from build123d import *

# Parameters (mm, degrees)
F1_DEPTH         = 17.5
F2_W             = 8
F2_H             = 3
F2_W_2           = 15
F2_H_2           = 1
F3_DEPTH         = 50
F5_DEPTH         = 2.5
F5_COPIES2_COUNT = 2


# Not quite as in the source:
# - a pattern or mirror of a feature is missing from the dataset's text; its kind, count and spacing are read off the source's solid


with BuildPart() as f1:
    # F0 (on Front) → F1 (new body, symmetric)
    with BuildSketch(Plane.XZ):
        Polygon((-11.8, 0), (0, 0), (11.8, 0), (11.8, 8), (11.5, 8), (8.5, 2.5), (0, 2.5), (-8.5, 2.5), (-11.5, 8), (-11.8, 8), align=None)
    extrude(amount=F1_DEPTH, both=True)

    # F2 (on Right) → F3 (cut, symmetric)
    with BuildSketch(Plane.YZ):
        with Locations((0, 4)):
            Rectangle(F2_W, F2_H)
        with Locations((0, 0.5)):
            Rectangle(F2_W_2, F2_H_2)
    extrude(amount=F3_DEPTH, both=True, mode=Mode.SUBTRACT)

    # F4 (on Top) → F5 (join)
    with BuildSketch(Plane.XY):
        Polygon((16, 18.5), (11.8, 17.5), (11.8, 7.5), (20, 15.5), (20, 31.5), (16, 31.5), align=None)
    f5 = extrude(amount=F5_DEPTH)

    # F5_copies: F5 across plane
    add(f5.mirror(Plane(origin=(0, 0, 0), x_dir=(0, 0, -1), z_dir=(-1, 0, 0))))

    # F5_copies1: F5 across plane
    add(f5.mirror(Plane(origin=(0, 0, 0), x_dir=(0, 0, -1), z_dir=(0, -1, 0))))

    # F5_copies2: F5 ×2 about axis
    f5_copies2_axis = Axis((0, 0, 0), (0, 0, 1))
    for i in range(1, F5_COPIES2_COUNT):
        add(f5.rotate(f5_copies2_axis, i * 360 / F5_COPIES2_COUNT))


solid = f1.part
Input: part model. Units: mm. Frame: model coordinates. A direction names the side the tool comes from. Give positions to 0.01 mm unless a question says otherwise; leave off trailing zeros. Order: outer loops, then holes, each group sorted by start corner. A loop starts at its lowest first (then second) coordinate and runs counter-clockwise, first axis right, second up. Notation, with made-up numbers: M -7,87 L 12,87 A18 ccw 12,107 Z; hole C 61,44.25 d8. An arc over 180 degrees is marked long. Answer as a JSON object with one key per item and string values.
1. Pull-direction query (Z, two-part tool) for faces 1 (the flat face through (18, 31.5, 1)), 2 (the flat face through (0, -17, 0)), 3 (the flat face through (10, 4, 4)); classes: +Z half, -Z half, draft (parallel to the pull), parting line (faces both ways), or undercut.
Result sheet:
{"face 1": "draft", "face 2": "-Z half", "face 3": "undercut"}
2. Cut plane A-A, the plane y = -26. Output: boundary loops of the cut face in (x, z), and give its area (3 significant figures).
Result sheet:
{"outline": "M -20,0 L -16,0 L -16,2.5 L -20,2.5 Z; M 16,0 L 20,0 L 20,2.5 L 16,2.5 Z", "area": "20.0 mm²"}
3. Cut plane B-B, the plane x = -14.5. Output: boundary loops of the cut face in (y, z), and give its area (3 significant figures).
Result sheet:
{"outline": "M -18.14,0 L -10.13,0 L -10.13,2.5 L -18.14,2.5 Z; M 10.13,0 L 18.14,0 L 18.14,2.5 L 10.13,2.5 Z", "area": "40.0 mm²"}
4. Reachability of faces 4 (the flat face through (17, 20, 2.5)), 5 (the flat face through (-17, -20, 2.5)), 6 (the flat face through (16, -25, 1)), 7 (the flat face through (-11, 4, 4)), 8 (the flat face through (13.9, 18, 1.2)) from +Z, -Z, +X, -X, +Y, -Y: full face, straight path, thin tool, end or side. Return the list, or none.
Result sheet:
{"face 4": "+Z, +X, +Y, -Y", "face 5": "+Z, -X, +Y, -Y", "face 6": "+Z, -Z, -Y", "face 7": "+X, -X", "face 8": "+Z, -Z, +Y"}
5. Ray query, line 1 (Y direction, x = 0, z = 0.5); line 2 (X direction, y = 7.5, z = 6); line 3 (X direction, y = -7, z = 1.25). Return the intervals inside material, ascending. Write a range as [from, to].
Result sheet:
{"line 1": "[-17.5, -7.5], [7.5, 17.5]", "line 2": "[-11.8, -10.41], [10.41, 11.8]", "line 3": "[-11.8, 11.8]"}
6. First-contact query: P1, Ø7, axis at x = 4.5, y = -6, coming from the +Z side; P2, Ø10, axis at x = 2.5, y = -1, coming from the -Z side; P3, Ø10, axis at x = 5.5, y = 10, coming from the -Z side; P4, Ø1.1, axis at x = -1, z = 0.5, coming from the +Y side. Flat tips, straight axial feed; report the tip coordinate or a pass-through.
Result sheet:
{"P1": "z = 2.5", "P2": "z = 1", "P3": "z = 0", "P4": "y = 17.5"}
7. Cut plane C-C, the plane z = 4. Output: boundary loops of the cut face in (x, y), and give its area (3 significant figures).
Result sheet:
{"outline": "M -11.8,-17.5 L -9.32,-17.5 L -9.32,-4 L -11.8,-4 Z; M -11.8,4 L -9.32,4 L -9.32,17.5 L -11.8,17.5 Z; M 9.32,-17.5 L 11.8,-17.5 L 11.8,-4 L 9.32,-4 Z; M 9.32,4 L 11.8,4 L 11.8,17.5 L 9.32,17.5 Z", "area": "134 mm²"}
8. Cut plane D-D, the plane x = 1.5. Output: boundary loops of the cut face in (y, z), and give its area (3 significant figures).
Result sheet:
{"outline": "M -17.5,0 L -7.5,0 L -7.5,1 L 7.5,1 L 7.5,0 L 17.5,0 L 17.5,2.5 L -17.5,2.5 Z", "area": "72.5 mm²"}
